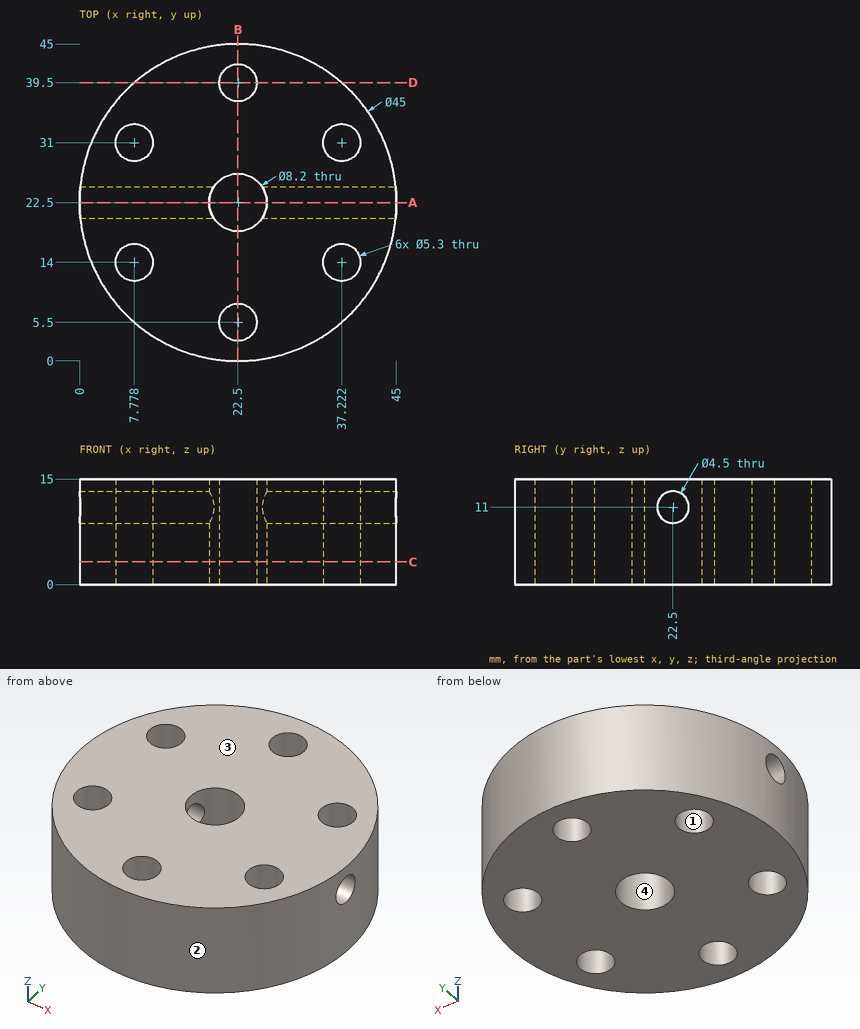
For this review, use the dimensioned drawing (mm, ordinates from the lowest corner) and the shaded views. Coordinates: 2 decimals unless noted, no trailing zeros. Order: outer loops, then holes, each group sorted by start corner. A loop starts at its lowest first (then second) coordinate and runs counter-clockwise, first axis right, second up. Notation, with made-up numbers: (33.25, -11.75) - (92.25, -11.75) arc R25 cw to (92.25, 23.25) - close; hole circle Ø5 at (49, 78). An arc over 180 degrees is marked (long way). Answer as a JSON object with one key per item and string values. Group by question number.
1. We need section C-C on z = 3.25. State the section outline as (x, y) points.
2. For probe 1 along Y at (x, z) = (22.5, 7.75); probe 2 along X at (y, z) = (20, 1); probe 3 along Z at (x, y) = (12, 22) (1 decimal), list the stretches that pass through material, from the lowest coordinate up.
3. The part is to be moulded in two halves that separate along X. For the marked faces 1, 2, 3 and 4, say which applies: pulls with the +X half, pulls with the -X half, needs draft (parallel to the pull), parting line crosses it, or undercut.
4. Clearance check with flat-ended pins moving along their axes: P1, Ø4, axis at y = 26, z = 10, coming from the +X side; P2, Ø3, axis at x = 12, z = 12, coming from the +Y side; P3, Ø2, axis at y = 10.5, z = 12, coming from the +X side. State where each tip first meets the part, or that it passes through.
5. We need section B-B on x = 22.5. State the section outline as (y, z) points, then the cut area to 3 significant figures.
6. We need section D-D on y = 39.5. State the section outline as (x, z) points.
7. We need section A-A on y = 22.5. State the section outline as (x, z) points.
Final values:
{
 "1": {"outline": "circle Ø45 at (22.5, 22.5); hole circle Ø5.3 at (7.78, 14); hole circle Ø5.3 at (7.78, 31); hole circle Ø8.2 at (22.5, 22.5); hole circle Ø5.3 at (22.5, 5.5); hole circle Ø5.3 at (22.5, 39.5); hole circle Ø5.3 at (37.22, 14); hole circle Ø5.3 at (37.22, 31)"},
 "2": {"probe 1": "0 to 2.85, 8.15 to 18.4, 26.6 to 36.85, 42.15 to 45", "probe 2": "0.14 to 19.25, 25.75 to 44.86", "probe 3": "0 to 8.8, 13.2 to 15"},
 "3": {"face 1": "undercut", "face 2": "parting line crosses it", "face 3": "needs draft", "face 4": "undercut"},
 "4": {"P1": "x = 44.94", "P2": "y = 43.12", "P3": "x = 42.13"},
 "5": {"outline": "(0, 0) - (2.85, 0) - (2.85, 15) - (0, 15) - close; (8.15, 0) - (18.4, 0) - (18.4, 15) - (8.15, 15) - close; (26.6, 0) - (36.85, 0) - (36.85, 15) - (26.6, 15) - close; (42.15, 0) - (45, 0) - (45, 15) - (42.15, 15) - close", "area": "393 mm²"},
 "6": {"outline": "(7.76, 0) - (19.85, 0) - (19.85, 15) - (7.76, 15) - close; (25.15, 0) - (37.24, 0) - (37.24, 15) - (25.15, 15) - close"},
 "7": {"outline": "(0, 0) - (18.4, 0) - (18.4, 8.75) - (0, 8.75) - close; (0, 13.25) - (18.4, 13.25) - (18.4, 15) - (0, 15) - close; (26.6, 0) - (45, 0) - (45, 8.75) - (26.6, 8.75) - close; (26.6, 13.25) - (45, 13.25) - (45, 15) - (26.6, 15) - close"}
}
